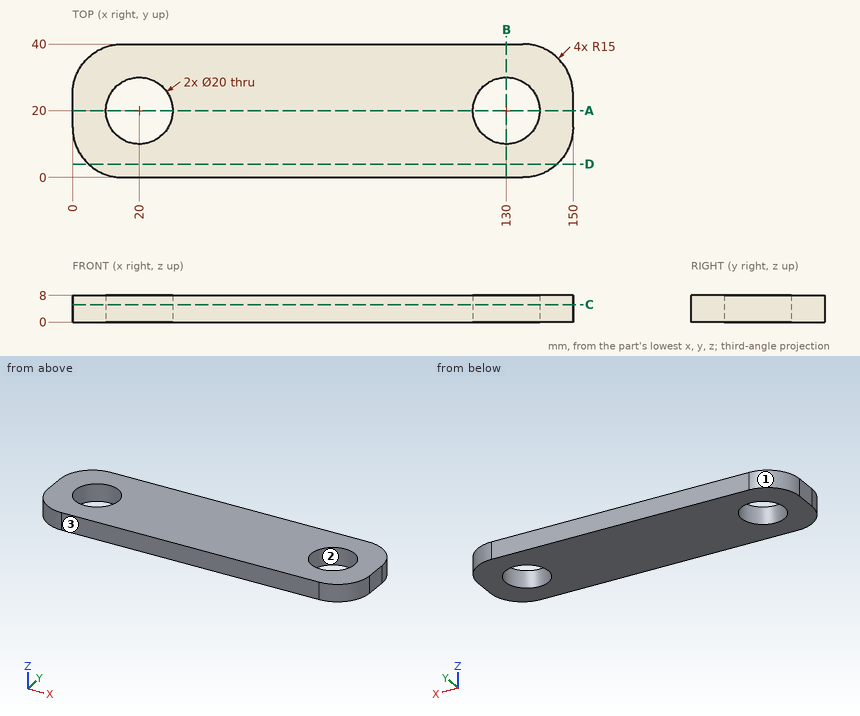
Print and shaded views of the part. All mm, measured from the part's lowest x, y and z. Give positions to 0.01 mm unless a question says otherwise; leave off trailing zeros. Loops run counter-clockwise (first coordinate to the right, second up) from the corner with the lowest first, then second, coordinate; pieces in that order, holes last. Notation, with made-up numbers: (-38.75, 22.25) -> (-11.75, 22.25) arc R21 ccw to (-11.75, 39.25) -> close; hole circle Ø2 at (16, -31). An arc over 180 degrees is marked (long way). Use a Markdown table: item, result.
1. Mould opens along X. For the marked faces 1, 2 and 3 say: pulls with the +X half, pulls with the -X half, needs draft (parallel to the pull), parting line crosses it, or undercut.
Check result:
| item | result |
|---|---|
| face 1 | pulls with the -X half |
| face 2 | undercut |
| face 3 | needs draft |
2. Slice it at D-D (y = 4). List the corners of the cut face in (x, z), plus the area to 3 significant figures.
Check result:
| item | result |
|---|---|
| outline | (4.8, 0) -> (145.2, 0) -> (145.2, 8) -> (4.8, 8) -> close |
| area | 1,120 mm^2 |
3. Wall check: L1, parallel to Y at x = 20, z = 4.75; L2, parallel to X at y = 14, z = 3.5; L3, parallel to X at y = 17, z = 6.75. Give the ranges that are in metal, low to high. Write a range as [from, to].
Check result:
| item | result |
|---|---|
| L1 | y = [0, 10], [30, 40] |
| L2 | x = [0.03, 12], [28, 122], [138, 149.97] |
| L3 | x = [0, 10.46], [29.54, 120.46], [139.54, 150] |
4. Flat gauge pin, fed straight in: pin 1 (18 mm diameter, centred on x = 20, y = 20, fed in from +Z). Where does the tip first touch, or does it go through?
Check result:
| item | result |
|---|---|
| pin 1 | passes through |
5. Slice it at B-B (x = 130). List the corners of the cut face in (y, z).
Check result:
| item | result |
|---|---|
| outline | (0, 0) -> (10, 0) -> (10, 8) -> (0, 8) -> close; (30, 0) -> (40, 0) -> (40, 8) -> (30, 8) -> close |
6. Slice it at A-A (y = 20). List the corners of the cut face in (x, z).
Check result:
| item | result |
|---|---|
| outline | (0, 0) -> (10, 0) -> (10, 8) -> (0, 8) -> close; (30, 0) -> (120, 0) -> (120, 8) -> (30, 8) -> close; (140, 0) -> (150, 0) -> (150, 8) -> (140, 8) -> close |
7. Slice it at C-C (z = 5.25). List the corners of the cut face in (x, y).
Check result:
| item | result |
|---|---|
| outline | (0, 15) arc R15 ccw to (15, 0) -> (135, 0) arc R15 ccw to (150, 15) -> (150, 25) arc R15 ccw to (135, 40) -> (15, 40) arc R15 ccw to (0, 25) -> close; hole circle Ø20 at (20, 20); hole circle Ø20 at (130, 20) |
